Design review of the part shown in the three views and the two pictorial views. Dimensions are in mm from the part's minimum x, y and z. A direction names the side the tool comes from. Give positions to 0.01 mm unless a question says otherwise; leave off trailing zeros. Order: outer loops, then holes, each group sorted by start corner. A loop starts at its lowest first (then second) coordinate and runs counter-clockwise, first axis right, second up.
Item 1: Consider section B-B (y = 4). Give the boundary of the cut face in (x, z).
Item 2: For probe 1 along X at (y, z) = (4, 1.3); probe 2 along Y at (x, z) = (8.5, 1); probe 3 along X at (y, z) = (6, 1.7), list the stretches that pass through material, from the lowest coordinate up.
Item 3: For P1, Ø2.5, axis at x = 10.5, y = 3, coming from the -Z side; P2, Ø1.3, axis at x = 8, y = 3.5, coming from the -Z side; P3, Ø2, axis at x = 7.9, y = 4, coming from the +Z side, all flat-tipped, find the tip position at first contact; note any pin that passes through.
Item 4: Consider section C-C (x = 3.9). Give the boundary of the cut face in (y, z), plus the area to 3 significant figures.
Item 5: Consider section D-D (z = 4.75). Give the boundary of the cut face in (x, y), plus the area to 3 significant figures.
Item 6: The part is to be moulded in two halves that separate along Y. For the marked faces 4, 5 and 6, say which applies: released by +Y, released by -Y, zero draft, split by the parting line, or undercut.
Item 7: Consider section A-A (z = 0.9). Give the boundary of the cut face in (x, y).
Item 8: Machinability: for the marked faces 1, 2 and 3, which of the approach directions +Z, -Z, +X, -X, +Y, -Y give a long, thin tool a straight path to every point of the face, cutting with its end or side? Answer none if there is none.
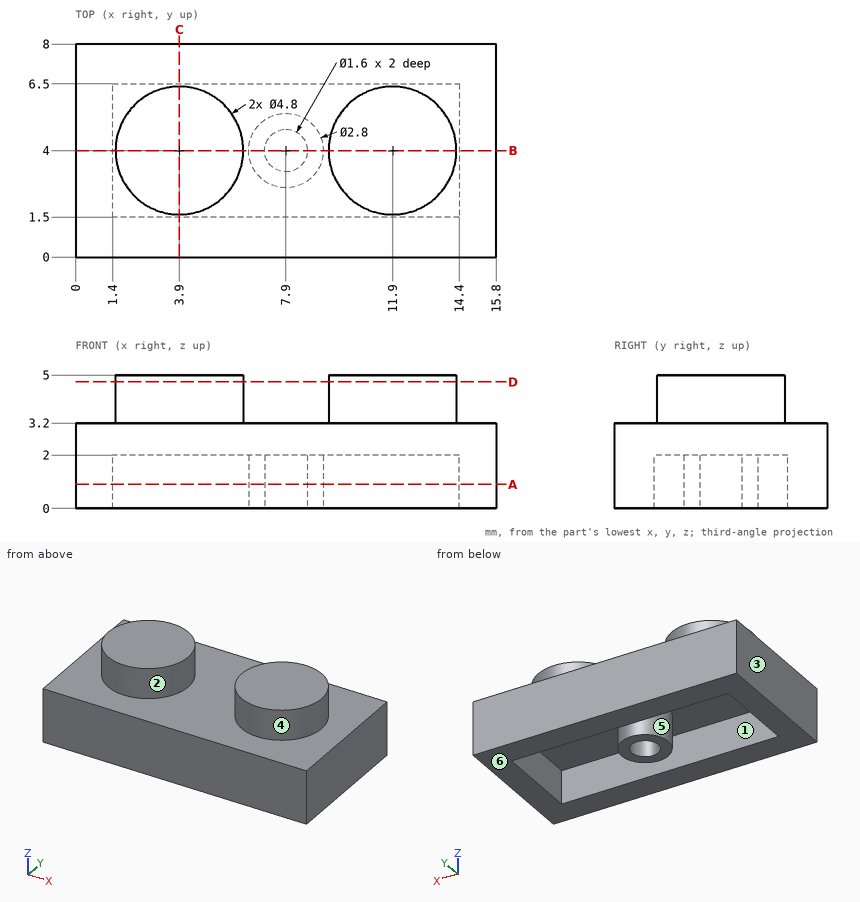
Resolved:
1. outline: (0, 0) - (1.4, 0) - (1.4, 2) - (6.5, 2) - (6.5, 0) - (7.1, 0) - (7.1, 2) - (8.7, 2) - (8.7, 0) - (9.3, 0) - (9.3, 2) - (14.4, 2) - (14.4, 0) - (15.8, 0) - (15.8, 3.2) - (14.3, 3.2) - (14.3, 5) - (9.5, 5) - (9.5, 3.2) - (6.3, 3.2) - (6.3, 5) - (1.5, 5) - (1.5, 3.2) - (0, 3.2) - close
2. probe 1: x = 0 to 1.4, 6.5 to 7.1, 8.7 to 9.3, 14.4 to 15.8
2. probe 2: y = 0 to 1.5, 2.74 to 3.47, 4.53 to 5.26, 6.5 to 8
2. probe 3: x = 0 to 1.4, 14.4 to 15.8
3. P1: stops at z = 2
3. P2: stops at z = 0
3. P3: stops at z = 3.2
4. outline: (0, 0) - (1.5, 0) - (1.5, 2) - (6.5, 2) - (6.5, 0) - (8, 0) - (8, 3.2) - (6.4, 3.2) - (6.4, 5) - (1.6, 5) - (1.6, 3.2) - (0, 3.2) - close
4. area: 24.2 mm2
5. outline: circle Ø4.8 at (3.9, 4); circle Ø4.8 at (11.9, 4)
5. area: 36.2 mm2
6. face 4: split by the parting line
6. face 5: undercut
6. face 6: zero draft
7. outline: (0, 0) - (15.8, 0) - (15.8, 8) - (0, 8) - close; circle Ø2.8 at (7.9, 4); hole (1.4, 1.5) - (14.4, 1.5) - (14.4, 6.5) - (1.4, 6.5) - close; hole circle Ø1.6 at (7.9, 4)
8. face 1: -Z
8. face 2: +Z
8. face 3: +Z, -Z, -X, +Y, -Y
